Answer from the drawing. Dimensions are ordinates in mm from the lowest x, y and z of the part. Round coordinates to 2 decimals unless told otherwise and drop trailing zeros. Loops run counter-clockwise (first coordinate to the right, second up) from the corner with the lowest first, then second, coordinate; pieces in that order, holes last. Notation, with made-up numbers: M -20,19.5 L -16,19.5 A24 cw -16,37.5 Z; hole C 46.25,64 d9. An arc over 180 degrees is marked long. Answer as CSV lines item,"result".
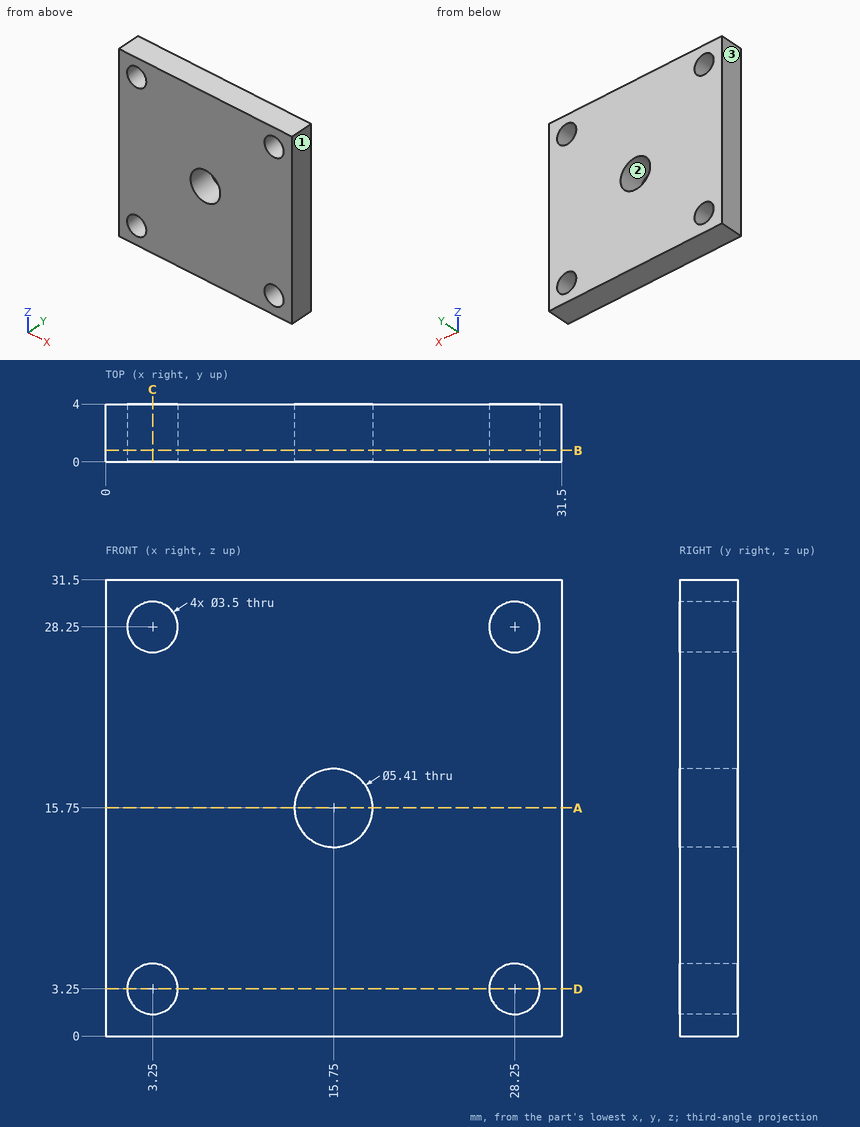
1) Determine the mould class of the marked faces 1, 2 and 3 for opening direction X: released by +X, released by -X, zero draft, split by the parting line, or undercut.
Evaluation:
face 1,"released by +X"
face 2,"undercut"
face 3,"released by -X"
2) Find section C-C, the plane x = 3.25. Give the vertices of the cut face in (y, z), then the cut area to 3 significant figures.
Evaluation:
outline,"M 0,0 L 4,0 L 4,1.5 L 0,1.5 Z; M 0,5 L 4,5 L 4,26.5 L 0,26.5 Z; M 0,30 L 4,30 L 4,31.5 L 0,31.5 Z"
area,"98.0 mm^2"
3) Find section D-D, the plane z = 3.25. Give the vertices of the cut face in (x, y), then the cut area to 3 significant figures.
Evaluation:
outline,"M 0,0 L 1.5,0 L 1.5,4 L 0,4 Z; M 5,0 L 26.5,0 L 26.5,4 L 5,4 Z; M 30,0 L 31.5,0 L 31.5,4 L 30,4 Z"
area,"98.0 mm^2"
4) Find section B-B, the plane y = 0.8. Count the separate pieces of the cut face and the enclosed holes in it, then the cut area to 3 significant figures.
Evaluation:
separate pieces,"1"
enclosed holes,"5"
area,"931 mm^2"
5) Each of these flat-tipped pins is pushed along its axis until it touches: P1, Ø8, axis at x = 18, z = 21, coming from the -Y side; P2, Ø3, axis at x = 28.25, z = 28.25, coming from the -Y side. Where does it stop, or does it pass through?
Evaluation:
P1,"stops at y = 0"
P2,"passes through"
6) Find section A-A, the plane z = 15.75. Give the vertices of the cut face in (x, y) (1 decimal).
Evaluation:
outline,"M 0,0 L 13,0 L 13,4 L 0,4 Z; M 18.5,0 L 31.5,0 L 31.5,4 L 18.5,4 Z"
7) Straight lines are drawn through the part: line 1 (Z direction, x = 3.25, y = 2.6); line 2 (Z direction, x = 4.5, y = 1.5) (1 decimal). For each, find the intervals that lie inside material, in ascending order.
Evaluation:
line 1,"z = 0 to 1.5, 5 to 26.5, 30 to 31.5"
line 2,"z = 0 to 2, 4.5 to 27, 29.5 to 31.5"
